Input: part model. Units: mm. Frame: model coordinates. Face numbers are marked on the shaded views. A direction names the side the tool comes from. Give positions to 0.01 mm unless a question says otherwise; leave off trailing zeros. Write each loop counter-clockwise with the first axis right and the second up, starting at its lowest first coordinate (ties: lowest second). Pieces come first, ordered by that corner, then holes. Notation, with made-up numbers: (-32, 52) - (12, 52) arc R25 ccw to (12, 75) - close; hole circle Ø5 at (42.5, 43). An arc over 180 degrees is marked (long way). Use a Markdown table: item, result. Add a question column.
1. Section query A-A, the plane x = -27. Return loops of the section in (y, z), plus the area to 3 significant figures.
2. Section query C-C, the plane y = 1.7. Return loops of the section in (x, z).
3. Pin query (flat end, axial travel): pin 1 (10 mm diameter, centred on x = -12, z = -25, fed in from -Y); pin 2 (1 mm diameter, centred on x = -32.5, y = 3, fed in from +Z); pin 3 (2.5 mm diameter, centred on x = -12.5, y = 3.5, fed in from -Z); pin 4 (1.5 mm diameter, centred on x = -5.5, y = 4, fed in from -Z). Return the tip coordinate at first contact, or that it passes through.
4. Mould query, pull axis X, two halves, no side actions, for the marked faces 1, 2, 3 and 4. Classes: released by +X, released by -X, zero draft, split by the parting line, or undercut.
5. Section query B-B, the plane z = -19.25. Return loops of the section in (x, y), plus the area to 3 significant figures.
6. Material intervals for probe 1 along X at (y, z) = (2.1, -19.25); probe 2 along X at (y, z) = (3.8, -9.75); probe 3 along X at (y, z) = (0.9, -10.5), sorted ascending.
7. Set-up query: the marked faces 5, 6 and 7. Return all of +Z, -Z, +X, -X, +Y, -Y with unobstructed straight access to the full face (end or side cutting, diameter ignored); none if empty.
8. Section query D-D, the plane x = -9. Return loops of the section in (y, z).
```python
from build123d import *

# Parameters (mm, degrees)
BOSS_EXTRUDE1_DEPTH = 5
SKETCH2_W           = 20
SKETCH2_H           = 5
BOSS_EXTRUDE2_DEPTH = 7.5
SKETCH3_W           = 20
SKETCH3_H           = 5
BOSS_EXTRUDE3_DEPTH = 5
CUT_EXTRUDE2_REACH  = 7
CUT_EXTRUDE3_REACH  = 7
SKETCH7_R           = 1
CUT_EXTRUDE4_REACH  = 7
SKETCH8_R           = 1


with BuildPart() as part:
    # Sketch1 → Boss-Extrude1 (new body)
    with BuildSketch(Plane(origin=(0, 0, 0), x_dir=(1, 0, 0), z_dir=(0, 1, 0))):
        Polygon((-37.172745284, 27.474605058), (-17.172745284, 27.474605058), (-1.172745284, 11.474605058), (-21.172745284, 11.474605058), align=None)
    extrude(amount=BOSS_EXTRUDE1_DEPTH)

    # Sketch2 → Boss-Extrude2 (add)
    with BuildSketch(Plane(origin=(0, 0, -27.474605058), x_dir=(-1, 0, 0), z_dir=(0, 0, -1))):
        with Locations((27.172745284, 2.5)):
            Rectangle(SKETCH2_W, SKETCH2_H)
    extrude(amount=BOSS_EXTRUDE2_DEPTH)

    # Sketch3 → Boss-Extrude3 (add)
    with BuildSketch(Plane.XY.offset(-11.474605058)):
        with Locations((-11.172745284, 2.5)):
            Rectangle(SKETCH3_W, SKETCH3_H)
    extrude(amount=BOSS_EXTRUDE3_DEPTH)

    # Sketch5 → Cut-Extrude2 (cut, up to next)
    with BuildSketch(Plane(origin=(0, 5, 0), x_dir=(1, 0, 0), z_dir=(0, 1, 0)), mode=Mode.PRIVATE) as cut_extrude2_sk1:
        Polygon((-16.784341734, 22.843560821), (-8.415385971, 14.474605058), (-18.876580675, 14.474605058), align=None)
    cut_extrude2_tool1 = extrude(cut_extrude2_sk1.sketch, amount=-CUT_EXTRUDE2_REACH, mode=Mode.PRIVATE) & part.part
    add(cut_extrude2_tool1.solids().sort_by_distance((-14.692103, 5, -17.264257))[0], mode=Mode.SUBTRACT)
    # Sketch5 → Cut-Extrude2 (cut, up to next)
    with BuildSketch(Plane(origin=(0, 5, 0), x_dir=(1, 0, 0), z_dir=(0, 1, 0)), mode=Mode.PRIVATE) as cut_extrude2_sk2:
        Polygon((-21.561148834, 16.105649296), (-29.930104597, 24.474605058), (-19.468909894, 24.474605058), align=None)
    cut_extrude2_tool2 = extrude(cut_extrude2_sk2.sketch, amount=-CUT_EXTRUDE2_REACH, mode=Mode.PRIVATE) & part.part
    add(cut_extrude2_tool2.solids().sort_by_distance((-23.653388, 5, -21.684953))[0], mode=Mode.SUBTRACT)

    # Sketch7 → Cut-Extrude3 (cut, up to next)
    with BuildSketch(Plane(origin=(0, 5, 0), x_dir=(1, 0, 0), z_dir=(0, 1, 0)), mode=Mode.PRIVATE) as cut_extrude3_sk1:
        with Locations((-15.172745284, 8.974605058)):
            Circle(SKETCH7_R)
    cut_extrude3_tool1 = extrude(cut_extrude3_sk1.sketch, amount=-CUT_EXTRUDE3_REACH, mode=Mode.PRIVATE) & part.part
    add(cut_extrude3_tool1.solids().sort_by_distance((-15.172745, 5, -8.974605))[0], mode=Mode.SUBTRACT)
    # Sketch7 → Cut-Extrude3 (cut, up to next)
    with BuildSketch(Plane(origin=(0, 5, 0), x_dir=(1, 0, 0), z_dir=(0, 1, 0)), mode=Mode.PRIVATE) as cut_extrude3_sk2:
        with Locations((-7.172745284, 8.974605058)):
            Circle(SKETCH7_R)
    cut_extrude3_tool2 = extrude(cut_extrude3_sk2.sketch, amount=-CUT_EXTRUDE3_REACH, mode=Mode.PRIVATE) & part.part
    add(cut_extrude3_tool2.solids().sort_by_distance((-7.172745, 5, -8.974605))[0], mode=Mode.SUBTRACT)

    # Sketch8 → Cut-Extrude4 (cut, up to next)
    with BuildSketch(Plane(origin=(0, 5, 0), x_dir=(1, 0, 0), z_dir=(0, 1, 0)), mode=Mode.PRIVATE) as cut_extrude4_sk1:
        with Locations((-21.472745284, 31.224605058)):
            Circle(SKETCH8_R)
    cut_extrude4_tool1 = extrude(cut_extrude4_sk1.sketch, amount=-CUT_EXTRUDE4_REACH, mode=Mode.PRIVATE) & part.part
    add(cut_extrude4_tool1.solids().sort_by_distance((-21.472745, 5, -31.224605))[0], mode=Mode.SUBTRACT)
    # Sketch8 → Cut-Extrude4 (cut, up to next)
    with BuildSketch(Plane(origin=(0, 5, 0), x_dir=(1, 0, 0), z_dir=(0, 1, 0)), mode=Mode.PRIVATE) as cut_extrude4_sk2:
        with Locations((-27.472745284, 31.224605058)):
            Circle(SKETCH8_R)
    cut_extrude4_tool2 = extrude(cut_extrude4_sk2.sketch, amount=-CUT_EXTRUDE4_REACH, mode=Mode.PRIVATE) & part.part
    add(cut_extrude4_tool2.solids().sort_by_distance((-27.472745, 5, -31.224605))[0], mode=Mode.SUBTRACT)


solid = part.part
```
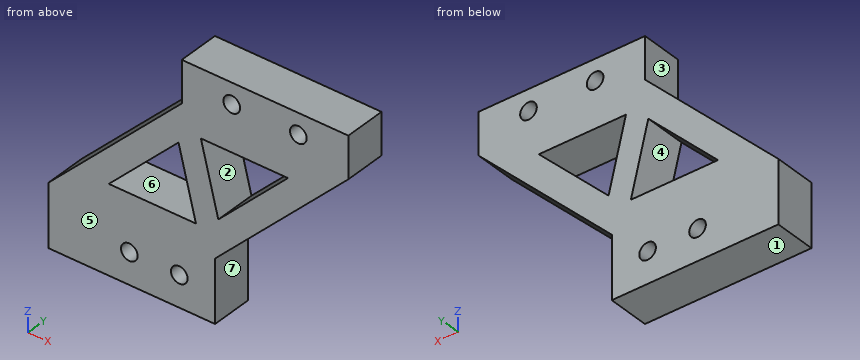
Result sheet:
| question | item | result |
|---|---|---|
| 1 | outline | (0, -34.97) - (5, -34.97) - (5, -32.11) - (0, -32.11) - close; (0, -30.34) - (5, -30.34) - (5, -24.47) - (0, -24.47) - close; (0, -21.54) - (5, -21.54) - (5, -17.3) - (0, -17.3) - close |
| 1 | area | 64.9 mm² |
| 2 | outline | (-37.17, -34.97) - (-17.17, -34.97) - (-17.17, -27.47) - (-1.17, -11.47) - (-1.17, -6.47) - (-21.17, -6.47) - (-21.17, -11.47) - (-37.17, -27.47) - close; hole (-29.93, -24.47) - (-19.47, -24.47) - (-21.56, -16.11) - close; hole circle Ø2 at (-27.47, -31.22); hole circle Ø2 at (-21.47, -31.22); hole (-18.88, -14.47) - (-16.78, -22.84) - (-8.42, -14.47) - close; hole circle Ø2 at (-15.17, -8.97); hole circle Ø2 at (-7.17, -8.97) |
| 3 | pin 1 | stops at y = 0 |
| 3 | pin 2 | stops at z = -22.3 |
| 3 | pin 3 | stops at z = -24.05 |
| 3 | pin 4 | stops at z = -16.55 |
| 4 | face 1 | zero draft |
| 4 | face 2 | undercut |
| 4 | face 3 | released by -X |
| 4 | face 4 | undercut |
| 5 | outline | (-28.95, 0) - (-24.71, 0) - (-24.71, 5) - (-28.95, 5) - close; (-20.78, 0) - (-17.68, 0) - (-17.68, 5) - (-20.78, 5) - close; (-13.19, 0) - (-8.95, 0) - (-8.95, 5) - (-13.19, 5) - close |
| 5 | area | 57.9 mm² |
| 6 | probe 1 | x = -28.95 to -24.71, -20.78 to -17.68, -13.19 to -8.95 |
| 6 | probe 2 | x = -21.17 to -15.8, -14.54 to -7.8, -6.54 to -1.17 |
| 6 | probe 3 | x = -21.17 to -1.17 |
| 7 | face 5 | +Z, -Z, +X, -X, -Y |
| 7 | face 6 | +Y, -Y |
| 7 | face 7 | -Z, +X, +Y, -Y |
| 8 | outline | (0, -19.3) - (5, -19.3) - (5, -15.06) - (0, -15.06) - close; (0, -14.47) - (5, -14.47) - (5, -6.47) - (0, -6.47) - close |
